Read the model definition and answer for the solid it produces. Units are mm, in the model's axes. Face numbers are marked on the shaded views. A direction names the side the tool comes from. Round coordinates to 2 decimals unless told otherwise and drop trailing zeros. Order: outer loops, then holes, each group sorted by start corner. A loop starts at its lowest first (then second) coordinate and runs counter-clockwise, first axis right, second up. Notation, with made-up numbers: (82.5, 51) -> (91.5, 51) arc R21 cw to (91.5, 59) -> close; hole circle Ø9 at (-32.75, 36.5). An arc over 180 degrees is marked (long way). Answer as a JSON object with one key per item and string values. Group by question number.
Item 1: Section D-D, the plane y = 31.5 is taken. Write down the section's boundary in (x, z).
Item 2: Section A-A, the plane y = 12.5 is taken. Write down the section's boundary in (x, z).
Item 3: For the marked faces 4 and 5, determine the directions among +Z, -Z, +X, -X, +Y, -Y from which every point of the face is accessible in a straight line to the end or side of a thin tool.
Item 4: The mould has two halves that part along Z. Classify the marked faces 1, 2 and 3: pulls with the +Z half, pulls with the -Z half, needs draft (parallel to the pull), parting line crosses it, or undercut.
Item 5: Consider probe 1 along Y at (x, z) = (-1.25, -1.4); probe 2 along Y at (x, z) = (0.5, -0.75); probe 3 along Z at (x, y) = (1.25, 3). Determine where each line is inside the solid, lowest interval first. Write a range as from..to.
Item 6: Section C-C, the plane x = -2.5 is taken. Write down the section's boundary in (y, z).
Item 7: Given P1, Ø1.5, axis at x = -0.5, z = -1.5, coming from the +Y side; P2, Ø1.8, axis at x = 0, z = 0, coming from the -Y side, each flat-ended and moving along its own axis, determine where each tip first touches the part or whether it passes through.
Item 8: Section B-B, the plane z = -2.2 is taken. Write down the section's boundary in (x, y).
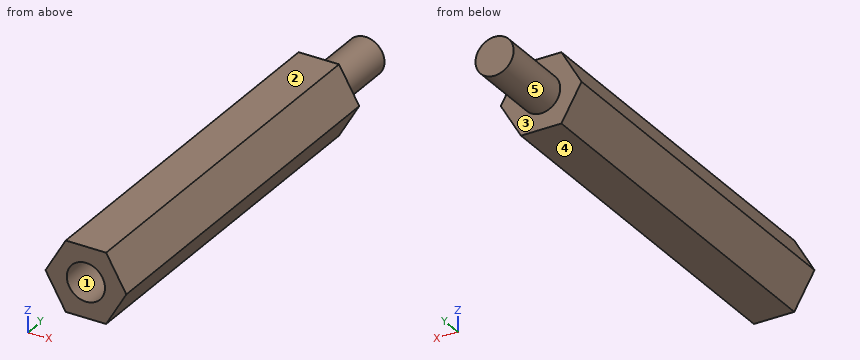
from build123d import *

# Parameters (mm, degrees)
BOSS_EXTRUDE1_DEPTH = 30
SKETCH2_R           = 1.5
CUT_EXTRUDE1_DEPTH  = 6
BOSS_EXTRUDE2_START = -30
SKETCH2_2_R         = 1.5
BOSS_EXTRUDE2_DEPTH = 6


with BuildPart() as part:
    # Sketch1 → Boss-Extrude1 (new body)
    with BuildSketch(Plane(origin=(0, 0, 0), x_dir=(1, 0, 0), z_dir=(0, 1, 0))):
        Polygon((1.58771324, -2.75), (3.175426481, 0), (1.58771324, 2.75), (-1.58771324, 2.75), (-3.175426481, 0), (-1.58771324, -2.75), align=None)
    extrude(amount=BOSS_EXTRUDE1_DEPTH)

    # Sketch2 → Cut-Extrude1 (cut)
    with BuildSketch(Plane.XZ):
        with Locations(Location((0, 0, 0), (0, 0, 270))):
            Circle(SKETCH2_R)
    extrude(amount=-CUT_EXTRUDE1_DEPTH, mode=Mode.SUBTRACT)

    # Sketch2<2> → Boss-Extrude2 (add)
    with BuildSketch(Plane.XZ.offset(BOSS_EXTRUDE2_START)):
        with Locations(Location((0, 0, 0), (0, 0, 270))):
            Circle(SKETCH2_2_R)
    extrude(amount=-BOSS_EXTRUDE2_DEPTH)


solid = part.part
Values found:
{
 "1": {"outline": "circle Ø3 at (0, 0)"},
 "2": {"outline": "(-3.18, 0) -> (-1.59, -2.75) -> (1.59, -2.75) -> (3.18, 0) -> (1.59, 2.75) -> (-1.59, 2.75) -> close"},
 "3": {"face 4": "-Z, +X, -X, +Y, -Y", "face 5": "+Y"},
 "4": {"face 1": "undercut", "face 2": "pulls with the +Z half", "face 3": "needs draft"},
 "5": {"probe 1": "0..30", "probe 2": "6..36", "probe 3": "-2.75..-0.83, 0.83..2.75"},
 "6": {"outline": "(0, -1.17) -> (30, -1.17) -> (30, 1.17) -> (0, 1.17) -> close"},
 "7": {"P1": "y = 36", "P2": "y = 6"},
 "8": {"outline": "(-1.91, 0) -> (1.91, 0) -> (1.91, 30) -> (-1.91, 30) -> close"}
}
